Autodesk Inventor part; units mm, degrees
ref_plane "YZ Plane" through (0, 0, 0) normal (1, 0, 0) x (0, 1, 0)
ref_plane "XZ Plane" through (0, 0, 0) normal (0, 1, 0) x (-1, 0, 0)
ref_plane "XY Plane" through (0, 0, 0) normal (0, 0, 1) x (1, 0, 0)
sketch "Sketch1" plane through (0, 0, 0) normal (0, 1, 0) x (-1, 0, 0)
  line L0 (0, 0) -> (130, 0)
  line L1 (130, 0) -> (130, -200)
  line L2 (130, -200) -> (0, -200)
  line L3 (0, -200) -> (0, 0)
  dimension "d0" = 130
  dimension "d1" = 200
extrude "Extrusion1" add sketch "Sketch1" along normal blind 25.4
sketch "Sketch2" plane through (0, 0, 0) normal (0, -1, 0) x (1, 0, 0)
  line L0 (0, -200) -> (-130, -200)
  line L1 (0, 0) -> (0, -200)
  line L2 (-102.952, -44.8611) -> (-27.048, -44.8611)
  line L3 (-27.048, -44.8611) -> (-27.048, -155.1389)
  line L4 (-27.048, -155.1389) -> (-102.952, -155.1389)
  line L5 (-102.952, -155.1389) -> (-102.952, -44.8611)
  line L6 (-102.952, -44.8611) -> (-27.048, -155.1389) construction
  line L7 (-27.048, -44.8611) -> (-102.952, -155.1389) construction
  line L8 (-130, -200) -> (-130, 0)
  line L9 (-130, 0) -> (0, 0)
  point P0 (-65, -100)
extrude "Extrusion2" add sketch "Sketch2" along normal blind 17.78
properties part number "Electronics place holder"
Read the model definition and answer for the solid it produces. Units are mm, in the model's axes. A direction names the side the tool comes from. Round coordinates to 2 decimals unless told otherwise and drop trailing zeros. Loops run counter-clockwise (first coordinate to the right, second up) from the corner with the lowest first, then second, coordinate; pieces in that order, holes last. Notation, with made-up numbers: (-10, -26) - (-2, -26) arc R32 ccw to (-2, 6) - close; hole circle Ø4 at (52.25, 26.25). An arc over 180 degrees is marked (long way). One line per question, with ' | ' between items. Start each with the question number.
Q1. For faces 1 (the flat face through (-64, 0, -99)), 2 (the flat face through (-66, 4, -200)), determine the directions among +Z, -Z, +X, -X, +Y, -Y from which every point of the face is accessible in a straight line to the end or side of a thin tool.
Q2. Section B-B on z = -120 is taken. Give the vertices of the cut face in (x, y).
Q3. For a pull along X with two mould halves and no side action, classify faces 3 (the flat face through (-109, -17.78, -99)), 4 (the flat face through (-27.048, -9, -99)), 5 (the flat face through (0, 4, -101)) as +X half, -X half, draft (parallel to the pull), parting line (faces both ways), or undercut.
Q4. Section C-C on y = -10 is taken. Give the vertices of the cut face in (x, z), plus the area to 3 significant figures.
Q5. Section A-A on x = -84.5 is taken. Give the vertices of the cut face in (y, z).
Q6. Flat-ended cylindrical pins translate along their axes: pin 1 (14 mm diameter, centred on y = -5.5, z = -87.5, fed in from +X); pin 2 (1.5 mm diameter, centred on x = -46, z = -75, fed in from -Y). Find the tip coordinate at first contact, or state that the pin passes through.
Q7. Find the intervals of material crossed by L1, parallel to X at y = -2, z = -110.5; L2, parallel to Z at x = -80.5, y = -10; L3, parallel to Y at x = -61.5, z = -106.5, in increasing order.
Established:
1) face 1: -Y | face 2: -Z, +X, -X, +Y, -Y
2) outline: (-130, -17.78) - (-102.95, -17.78) - (-102.95, 0) - (-27.05, 0) - (-27.05, -17.78) - (0, -17.78) - (0, 25.4) - (-130, 25.4) - close
3) face 3: draft | face 4: undercut | face 5: +X half
4) outline: (-130, -200) - (0, -200) - (0, 0) - (-130, 0) - close; hole (-102.95, -155.14) - (-27.05, -155.14) - (-27.05, -44.86) - (-102.95, -44.86) - close | area: 17,600 mm²
5) outline: (-17.78, -200) - (25.4, -200) - (25.4, 0) - (-17.78, 0) - (-17.78, -44.86) - (0, -44.86) - (0, -155.14) - (-17.78, -155.14) - close
6) pin 1: x = 0 | pin 2: y = 0
7) L1: -130 to -102.95, -27.05 to 0 | L2: -200 to -155.14, -44.86 to 0 | L3: 0 to 25.4
